```python
from build123d import *

# Parameters (mm, degrees)
SKIZZE1_R                       = 22.45
SKIZZE1_W                       = 30.1
SKIZZE1_H                       = 30.1
AUFSATZ_LINEAR_AUSTRAGEN1_DEPTH = 100
VERRUNDUNG1_R                   = 1
FASE1_SIZE                      = 2


with BuildPart() as part:
    # Skizze1 → Aufsatz-Linear austragen1 (new body)
    with BuildSketch(Plane.XY):
        Circle(SKIZZE1_R)
        Rectangle(SKIZZE1_W, SKIZZE1_H, mode=Mode.SUBTRACT)
    extrude(amount=AUFSATZ_LINEAR_AUSTRAGEN1_DEPTH)

    # Verrundung1
    verrundung1_edges = [part.edges().sort_by_distance(p)[0] for p in [
        (15.05, -15.05, 50),
        (15.05, 15.05, 50),
        (-15.05, 15.05, 50),
        (-15.05, -15.05, 50),
    ]]
    fillet(verrundung1_edges, radius=VERRUNDUNG1_R)

    # Fase1
    # the kernel refuses this chamfer: 2 mm, written as the material it takes off along each edge
    with BuildSketch(Plane(origin=(-15.05, -14.05, 0), x_dir=(-0.9996219169112968, 0, -0.02749587661058639), z_dir=(0, 1, 0)), Plane(origin=(14.05, -15.05, 0), x_dir=(0, -0.9996219169112968, -0.027495876610586424), z_dir=(-1, 0, 0)), Plane(origin=(15.05, 14.05, 0), x_dir=(0.9996219169112968, 0, -0.02749587661058639), z_dir=(0, -1, 0))) as fase1_piece_1:
        Polygon((FASE1_SIZE * 0.999621916911, FASE1_SIZE * 0.0274958766106), (-FASE1_SIZE * 0.0274958766106, FASE1_SIZE * 0.999621916911), (0, 0), align=None)
    extrude(amount=28.1, mode=Mode.SUBTRACT)
    with BuildSketch(Plane(origin=(-14.05, 15.05, 0), x_dir=(0, -0.027495876610586494, 0.9996219169112968), z_dir=(1, 0, 0))) as fase1_piece_2:
        Polygon((FASE1_SIZE * 0.999621916911, -FASE1_SIZE * 0.0274958766106), (-FASE1_SIZE * 0.0274958766106, -FASE1_SIZE * 0.999621916911), (0, 0), align=None)
    extrude(amount=28.1, mode=Mode.SUBTRACT)
    with BuildSketch(Plane(origin=(-14.05, -14.05, 0), x_dir=(0, -1, 0), z_dir=(1, 0, 0))) as fase1_piece_3:
        Polygon((1 + FASE1_SIZE, 0), (1, -FASE1_SIZE), (1, 0), align=None)
    revolve(axis=Axis((-14.05, -14.05, 0), (0, 0, -1)), revolution_arc=90, mode=Mode.SUBTRACT)
    with BuildSketch(Plane(origin=(14.05, -14.05, 0), x_dir=(1, 0, 0), z_dir=(0, 1, 0))) as fase1_piece_4:
        Polygon((1 + FASE1_SIZE, 0), (1, -FASE1_SIZE), (1, 0), align=None)
    revolve(axis=Axis((14.05, -14.05, 0), (0, 0, -1)), revolution_arc=90, mode=Mode.SUBTRACT)
    with BuildSketch(Plane(origin=(14.05, 14.05, 0), x_dir=(0, 1, 0), z_dir=(-1, 0, 0))) as fase1_piece_5:
        Polygon((1 + FASE1_SIZE, 0), (1, -FASE1_SIZE), (1, 0), align=None)
    revolve(axis=Axis((14.05, 14.05, 0), (0, 0, -1)), revolution_arc=90, mode=Mode.SUBTRACT)
    with BuildSketch(Plane(origin=(-14.05, 14.05, 0), x_dir=(0, 1, 0), z_dir=(1, 0, 0))) as fase1_piece_6:
        Polygon((1 + FASE1_SIZE, 0), (1, FASE1_SIZE), (1, 0), align=None)
    revolve(axis=Axis((-14.05, 14.05, 0), (0, 0, 1)), revolution_arc=90, mode=Mode.SUBTRACT)


solid = part.part
```
Design review of the part built by this model. Coordinates are the model's own, in mm. A direction names the side the tool comes from. Round coordinates to 2 decimals unless told otherwise and drop trailing zeros. Order: outer loops, then holes, each group sorted by start corner. A loop starts at its lowest first (then second) coordinate and runs counter-clockwise, first axis right, second up. Notation, with made-up numbers: (5.25, 16) - (37.25, 16) arc R20 ccw to (37.25, 54) - close; hole circle Ø10 at (62.5, 44.5). An arc over 180 degrees is marked (long way). Return JSON: item names as keys, results as strings.
Q1. Wall thickness on L1, parallel to X at y = 8, z = 86.5; L2, parallel to Y at x = 0, z = 87.5; L3, parallel to Y at x = 14, z = 59: over which ranges is each line inside the solid? List them lowest first. Write a range as [from, to].
Computed values:
{"L1": "x = [-20.98, -15.05], [15.05, 20.98]", "L2": "y = [-22.45, -15.05], [15.05, 22.45]", "L3": "y = [-17.55, -15.05], [15.05, 17.55]"}
Q2. The part is to be moulded in two halves that separate along Y. For faces 4 (the flat face through (0, 19, 0)), 5 (the cylindrical face through (-16.55, 15.17, 49.3)), 6 (the conical face through (-15.28, -15.31, 1.24)), say which applies: pulls with the +Y half, pulls with the -Y half, needs draft (parallel to the pull), parting line crosses it, or undercut.
Computed values:
{"face 4": "needs draft", "face 5": "parting line crosses it", "face 6": "undercut"}
Q3. Machinability: for faces 1 (the flat face through (-15.05, 0, 50)), 2 (the flat face through (16.06, 0.2, 0.99)), 3 (the flat face through (-19, 0, 0)), which of the approach directions +Z, -Z, +X, -X, +Y, -Y give a long, thin tool a straight path to every point of the face, cutting with its end or side? Answer none if there is none.
Computed values:
{"face 1": "+Z, -Z", "face 2": "-Z", "face 3": "-Z, +X, -X, +Y, -Y"}
Q4. Consider section A-A on y = 0. Write out the cut boundary in (x, z), plus the area to 3 significant figures.
Computed values:
{"outline": "(-22.45, 0) - (-17.05, 0) - (-15.05, 2) - (-15.05, 100) - (-22.45, 100) - close; (15.05, 2) - (17.05, 0) - (22.45, 0) - (22.45, 100) - (15.05, 100) - close", "area": "1,480 mm2"}
Q5. Consider section C-C on z = 76. Write out the cut boundary in (x, y).
Computed values:
{"outline": "circle Ø44.9 at (0, 0); hole (-15.05, -14.05) arc R1 ccw to (-14.05, -15.05) - (14.05, -15.05) arc R1 ccw to (15.05, -14.05) - (15.05, 14.05) arc R1 ccw to (14.05, 15.05) - (-14.05, 15.05) arc R1 ccw to (-15.05, 14.05) - close"}
Q6. For pin 1 Ø10 at (y, z) = (-12, 87) entering from +X; pin 2 Ø10 at (x, z) = (-16.5, 24.5) entering from +Y; pin 3 Ø2 at (x, z) = (-10.5, 53) entering from +Y, all flat-tipped, find the tip position at first contact; note any pin that passes through.
Computed values:
{"pin 1": "stops at x = 21.33", "pin 2": "stops at y = 19.28", "pin 3": "stops at y = 20.34"}
